Input: part model. Units: mm. Frame: model coordinates. Face numbers are marked on the shaded views. Coordinates: 2 decimals unless noted, no trailing zeros. Write each loop counter-clockwise with the first axis right and the second up, starting at its lowest first coordinate (ties: lowest second). Pieces come first, ordered by that corner, then holes. Notation, with made-up numbers: M 30,-22.5 L 67,-22.5 A12 ccw 67,-9.5 Z; hole C 18.5,1 d9. An arc over 180 degrees is marked long. Write each question's results on one line, items separated by ' | '. Start each with the question number.
1. Section query D-D, the plane y = 36. Output: boundary loops of the cut face in (x, z), and give its area (3 significant figures).
2. Ray query, probe 1 along Y at (x, z) = (0, 2.2); probe 2 along Y at (x, z) = (-0.75, 4.5); probe 3 along X at (y, z) = (10, 3.05). Return the intervals inside material, ascending.
3. First-contact query: pin 1 (4 mm diameter, centred on x = 0, y = 38.1, fed in from +Z). Flat tip, straight axial feed; report the tip coordinate or a pass-through.
4. Section query A-A, the plane y = 12.7. Output: boundary loops of the cut face in (x, z).
5. Pull-direction query (Y, two-part tool) for the marked faces 1, 2, 3 and 4; classes: +Y half, -Y half, draft (parallel to the pull), parting line (faces both ways), or undercut.
6. Section query C-C, the plane z = 3.6. Output: boundary loops of the cut face in (x, y), and give its area (3 significant figures).
7. Section query B-B, the plane x = 0. Output: boundary loops of the cut face in (y, z).
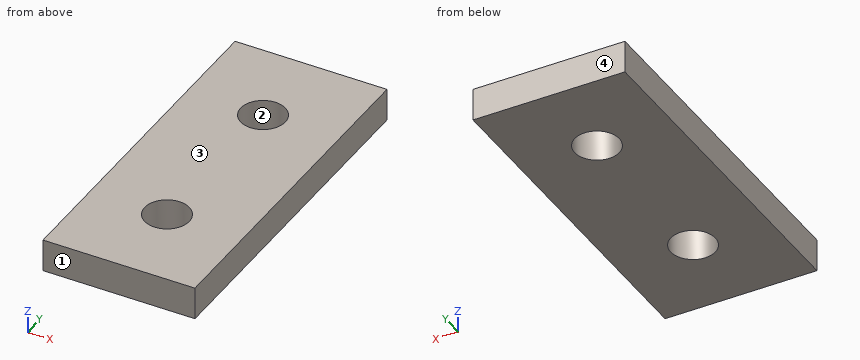
Autodesk Inventor part; units mm, degrees
ref_plane "YZ Plane" through (0, 0, 0) normal (1, 0, 0) x (0, 1, 0)
ref_plane "XZ Plane" through (0, 0, 0) normal (0, 1, 0) x (-1, 0, 0)
ref_plane "XY Plane" through (0, 0, 0) normal (0, 0, 1) x (1, 0, 0)
sketch "Sketch_1" plane through (0, 0, 0) normal (0, 0, 1) x (1, 0, 0)
  line L0 (-11.1125, 50.8) -> (-11.1125, 0)
  line L1 (-11.1125, 0) -> (11.1125, 0)
  line L2 (11.1125, 0) -> (11.1125, 50.8)
  line L3 (11.1125, 50.8) -> (-11.1125, 50.8)
  circle A0 centre (0, 12.7) radius 3.2639
  circle A1 centre (0, 38.1) radius 3.2639
extrude "Extrusion1" add sketch "Sketch_1" along normal blind 4.7752
properties part number "4107"
Answer:
1) outline: M -11.11,0 L -2.5,0 L -2.5,4.78 L -11.11,4.78 Z; M 2.5,0 L 11.11,0 L 11.11,4.78 L 2.5,4.78 Z | area: 82.3 mm^2
2) probe 1: 0 to 9.44, 15.96 to 34.84, 41.36 to 50.8 | probe 2: 0 to 9.52, 15.88 to 34.92, 41.28 to 50.8 | probe 3: -11.11 to -1.83, 1.83 to 11.11
3) pin 1: through
4) outline: M -11.11,0 L -3.26,0 L -3.26,4.78 L -11.11,4.78 Z; M 3.26,0 L 11.11,0 L 11.11,4.78 L 3.26,4.78 Z
5) face 1: -Y half | face 2: undercut | face 3: draft | face 4: +Y half
6) outline: M -11.11,0 L 11.11,0 L 11.11,50.8 L -11.11,50.8 Z; hole C 0,12.7 d6.53; hole C 0,38.1 d6.53 | area: 1,060 mm^2
7) outline: M 0,0 L 9.44,0 L 9.44,4.78 L 0,4.78 Z; M 15.96,0 L 34.84,0 L 34.84,4.78 L 15.96,4.78 Z; M 41.36,0 L 50.8,0 L 50.8,4.78 L 41.36,4.78 Z
